```python
from build123d import *

# Parameters (mm, degrees)
BASPROSKE_W        = 132.288
BASPROSKE_H        = 12
TOOTHCUT_DEPTH     = 134.372092073
TEETHCUTS_COUNT    = 10
TEETHCUTS_ANGLE    = 324
BORSKE_R           = 0.4
BORE_DEPTH         = 50.0000508
SKETCH1_R          = 15.199839534
SKETCH1_R_2        = 11.537985571
CUT_EXTRUDE1_DEPTH = 134.327124963
SCALE1_SCALE       = 0.4


with BuildPart() as part:
    # BasProSke → Base-Revolve (revolve)
    with BuildSketch(Plane(origin=(0, 0, 0), x_dir=(1, 0, 0), z_dir=(0, 1, 0)), mode=Mode.PRIVATE) as base_revolve_sk:
        with Locations((66.144, 6)):
            Rectangle(BASPROSKE_W, BASPROSKE_H)
    revolve(base_revolve_sk.sketch.rotate(Axis((-10, 0, 0), (1, 0, 0)), 180), axis=Axis((-10, 0, 0), (1, 0, 0)))

    # TooCutSke → ToothCut (cut, through all)
    with BuildSketch(Plane(origin=(0, 0, 0), x_dir=(0, 0, -1), z_dir=(1, 0, 0))):
        with BuildLine():
            ThreePointArc((1.173662691, 7.406586048), (0, 7.499), (-1.173662691, 7.406586048))
            ThreePointArc((-1.173662691, 7.406586048), (-1.668191438, 9.834565786), (-3.497907776, 11.50542856))
            ThreePointArc((-3.497907776, 11.50542856), (0, 12.0254), (3.497907776, 11.50542856))
            ThreePointArc((3.497907776, 11.50542856), (1.668191438, 9.834565786), (1.173662691, 7.406586048))
        make_face()
    toothcut = extrude(amount=TOOTHCUT_DEPTH, mode=Mode.SUBTRACT)

    # TeethCuts: ToothCut ×10 about axis
    teethcuts_axis = Axis((-10, 0, 0), (1, 0, 0))
    for i in range(1, TEETHCUTS_COUNT):
        add(toothcut.rotate(teethcuts_axis, i * TEETHCUTS_ANGLE / (TEETHCUTS_COUNT - 1)), mode=Mode.SUBTRACT)

    # BorSke → Bore (cut, symmetric)
    with BuildSketch(Plane(origin=(0, 0, 0), x_dir=(0, 0, -1), z_dir=(1, 0, 0))):
        Circle(BORSKE_R)
    extrude(amount=BORE_DEPTH, both=True, mode=Mode.SUBTRACT)

    # Sketch1 → Cut-Extrude1 (cut, through all)
    with BuildSketch(Plane(origin=(132.288, 0, 0), x_dir=(0, 0, -1), z_dir=(1, 0, 0))):
        Circle(SKETCH1_R)
        Circle(SKETCH1_R_2, mode=Mode.SUBTRACT)
    extrude(amount=-CUT_EXTRUDE1_DEPTH, mode=Mode.SUBTRACT)


with BuildPart() as part_1:
    # Scale1: scaled about (0, 0, 0)
    add(part.part.scale(SCALE1_SCALE))


solid = part_1.part
```
The listing builds one solid part. Answer for the finished solid, in the listing's coordinates (mm). Give positions to 0.01 mm unless a question says otherwise; leave off trailing zeros. Order: outer loops, then holes, each group sorted by start corner. A loop starts at its lowest first (then second) coordinate and runs counter-clockwise, first axis right, second up. Notation, with made-up numbers: (-6, 62.5) - (15, 62.5) arc R22 cw to (15, 77.5) - close; hole circle Ø2 at (59, 35.25). An arc over 180 degrees is marked (long way). Answer in a Markdown table with one row per item. Add a question column.
Q1. Find the intervals of material crossed by line 1 along Y through (x, z) = (2.5, 1.5); line 2 along Y through (x, z) = (2, 0); line 3 along Z through (x, y) = (50, -2.25), in increasing order. Write a range as [from, to].
Q2. For a pull along Y with two mould halves and no side action, classify faces 1 (the flat face through (0, 1, 0)), 2 (the cylindrical face through (26.09, -0.93, -2.85)) as released by +Y, released by -Y, zero draft, split by the parting line, or undercut.
Q3. The part is cut by section A-A (y = 3.5). Determine the outline of the cut face in (x, z).
Q4. Given P1, Ø2, axis at x = 23.5, z = -3, coming from the +Y side; P2, Ø1.5, axis at x = 8.5, z = 0, coming from the -Y side, each flat-ended and moving along its own axis, determine where each tip first touches the part or whether it passes through.
Determined:
| question | item | result |
|---|---|---|
| 1 | line 1 | y = [-4.36, -2.85], [-2.6, 2.6], [2.85, 4.36] |
| 1 | line 2 | y = [-3, -0.16], [0.16, 3] |
| 1 | line 3 | z = [-3.8, -2.2], [-1.98, 1.98], [2.2, 3.8] |
| 2 | face 1 | zero draft |
| 2 | face 2 | undercut |
| 3 | outline | (0, -1.76) - (52.92, -1.76) - (52.92, -0.5) - (0, -0.5) - close; (0, 0.5) - (52.92, 0.5) - (52.92, 1.76) - (0, 1.76) - close |
| 4 | P1 | stops at y = 2.93 |
| 4 | P2 | stops at y = -4.06 |
